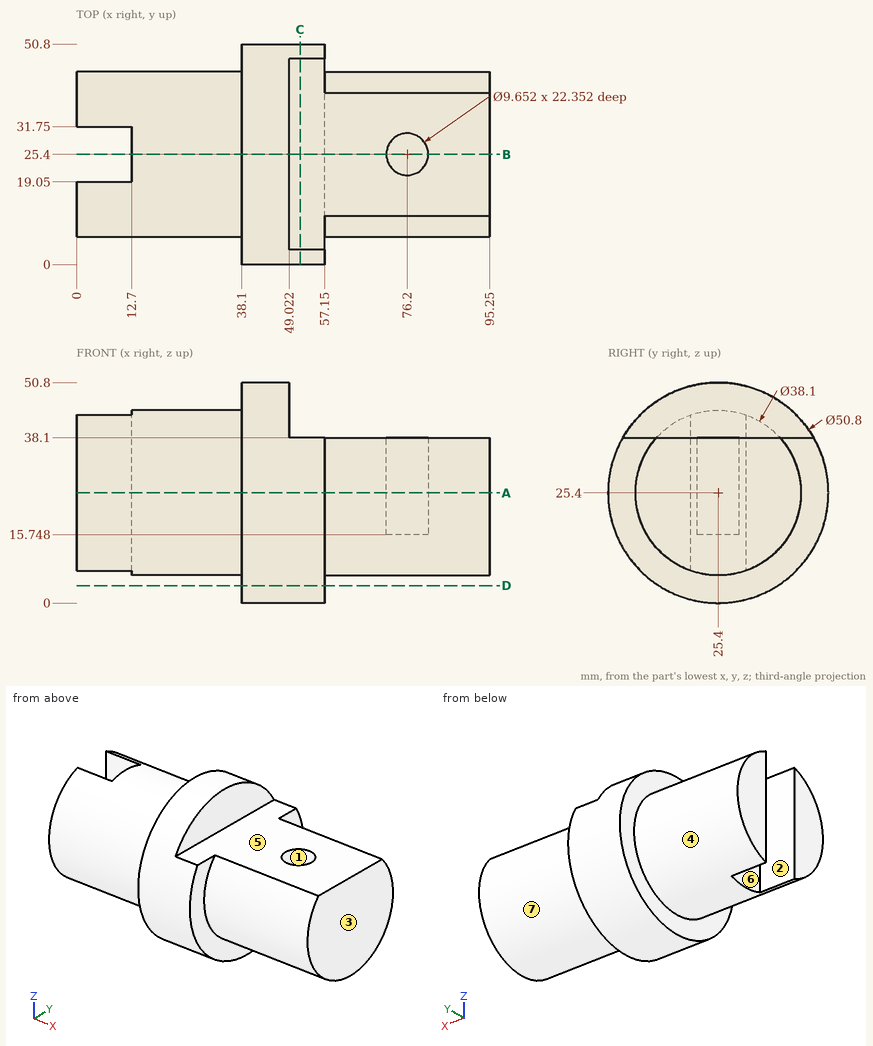
Answer from the drawing. Dimensions are ordinates in mm from the lowest x, y and z of the part. A direction names the side the tool comes from. Give positions to 0.01 mm unless a question says otherwise; leave off trailing zeros. Write each loop counter-clockwise with the first axis right and the second up, starting at its lowest first coordinate (ties: lowest second). Pieces come first, ordered by that corner, then holes. Notation, with made-up numbers: (66, 0.5) -> (87, 0.5) arc R17 cw to (87, 19.5) -> close; hole circle Ø7 at (60, 43). An arc over 180 degrees is marked (long way). Use a Markdown table: item, result.
(1) Find the intervals of material crossed by probe 1 along X at (y, z) = (25, 30); probe 2 along Y at (x, z) = (76.2, 33); probe 3 along Y at (x, z) = (10.5, 39.5), in increasing order. Write a range as from..to.
Return value:
| item | result |
|---|---|
| probe 1 | 12.7..71.39, 81.01..95.25 |
| probe 2 | 7.93..20.57, 30.23..42.87 |
| probe 3 | 12.59..19.05, 31.75..38.21 |
(2) Flat-ended cylindrical pins translate along their axes: P1, Ø4, axis at x = 82, z = 34.5, coming from the +Y side; P2, Ø14, axis at x = 8.5, z = 24, coming from the +Y side; P3, Ø4, axis at y = 15.5, z = 46.5, coming from the +X side. Find the tip coordinate at first contact, or state that the pin passes through.
Return value:
| item | result |
|---|---|
| P1 | y = 43.08 |
| P2 | y = 44.45 |
| P3 | x = 49.02 |
(3) For the marked faces 4, 5, 6 and 7, determine the directions among +Z, -Z, +X, -X, +Y, -Y from which every point of the face is accessible in a straight line to the end or side of a thin tool.
Return value:
| item | result |
|---|---|
| face 4 | -X |
| face 5 | +Z, +X, +Y, -Y |
| face 6 | +Z, -Z, -X |
| face 7 | +X |
(4) Determine the mould class of the marked faces 1, 2 and 3 for opening direction X: released by +X, released by -X, zero draft, split by the parting line, or undercut.
Return value:
| item | result |
|---|---|
| face 1 | undercut |
| face 2 | zero draft |
| face 3 | released by +X |
(5) Section B-B, the plane y = 25.4 is taken. Determine the outline of the cut face in (x, z), then the cut area to 3 significant figures.
Return value:
| item | result |
|---|---|
| outline | (12.7, 6.35) -> (38.1, 6.35) -> (38.1, 0) -> (57.15, 0) -> (57.15, 6.35) -> (95.25, 6.35) -> (95.25, 38.1) -> (81.03, 38.1) -> (81.03, 15.75) -> (71.37, 15.75) -> (71.37, 38.1) -> (49.02, 38.1) -> (49.02, 50.8) -> (38.1, 50.8) -> (38.1, 44.45) -> (12.7, 44.45) -> close |
| area | 2,830 mm2 |
(6) Section D-D, the plane z = 4 is taken. Determine the outline of the cut face in (x, y), then the cut area to 3 significant figures.
Return value:
| item | result |
|---|---|
| outline | (38.1, 11.72) -> (57.15, 11.72) -> (57.15, 39.08) -> (38.1, 39.08) -> close |
| area | 521 mm2 |
(7) Section A-A, the plane z = 25.4 is taken. Determine the outline of the cut face in (x, y).
Return value:
| item | result |
|---|---|
| outline | (0, 6.35) -> (38.1, 6.35) -> (38.1, 0) -> (57.15, 0) -> (57.15, 6.35) -> (95.25, 6.35) -> (95.25, 44.45) -> (57.15, 44.45) -> (57.15, 50.8) -> (38.1, 50.8) -> (38.1, 44.45) -> (0, 44.45) -> (0, 31.75) -> (12.7, 31.75) -> (12.7, 19.05) -> (0, 19.05) -> close; hole circle Ø9.65 at (76.2, 25.4) |
(8) Section C-C, the plane x = 51.5 is taken. Determine the outline of the cut face in (y, z).
Return value:
| item | result |
|---|---|
| outline | (3.4, 38.1) arc R25.4 ccw (long way) to (47.4, 38.1) -> close |
